from build123d import *

# Parameters (mm, degrees)
SKETCH_1_W             = 85
SKETCH_1_H             = 16
SKETCH_1_R             = 4.25
EXTRUDE_1_DEPTH        = 10
HOLE_WIZARD_M5_1_D     = 4.2
HOLE_WIZARD_M5_1_DEPTH = 14.9
HOLE_WIZARD_M5_1_TIP   = 1.2618073


with BuildPart() as part:
    # 草图1 → 凸台-拉伸1 (new body)
    with BuildSketch(Plane.XY):
        Rectangle(SKETCH_1_W, SKETCH_1_H)
        with Locations((-23, 0)):
            Circle(SKETCH_1_R, mode=Mode.SUBTRACT)
        with Locations((23, 0)):
            Circle(SKETCH_1_R, mode=Mode.SUBTRACT)
    extrude(amount=EXTRUDE_1_DEPTH)

    # M5 螺纹孔1
    with Locations(Plane.XY.offset(10)):
        with Locations((-35, 0), (35, 0)):
            Hole(HOLE_WIZARD_M5_1_D / 2, depth=HOLE_WIZARD_M5_1_DEPTH)
            with Locations((0, 0, -(HOLE_WIZARD_M5_1_DEPTH + HOLE_WIZARD_M5_1_TIP / 2))):  # 118° drill point
                Cone(0, HOLE_WIZARD_M5_1_D / 2, HOLE_WIZARD_M5_1_TIP, mode=Mode.SUBTRACT)


solid = part.part
Read the model definition and answer for the solid it produces. Units are mm, in the model's axes. Give positions to 0.01 mm unless a question says otherwise; leave off trailing zeros. Write each loop counter-clockwise with the first axis right and the second up, starting at its lowest first coordinate (ties: lowest second). Pieces come first, ordered by that corner, then holes. Notation, with made-up numbers: (28, 61.5) -> (44, 61.5) arc R12 ccw to (44, 71.5) -> close; hole circle Ø6 at (69, 34). An arc over 180 degrees is marked (long way). Answer as a JSON object with one key per item and string values. Group by question number.
1) Find section D-D (x = -35). Write down the section's boundary in (y, z), and give its area (3 significant figures).
2) The mould has two halves that part along X. Classify faces 1 (the flat face through (-1, 8, 5)), 2 (the flat face through (42.5, 0, 5)), 3 (the cylindrical face through (19.868, 2.872, 4.93)): +X half, -X half, draft (parallel to the pull), parting line (faces both ways), or undercut.
3) Find section A-A (y = 0). Write down the section's boundary in (x, z).
4) Find section B-B (x = 23). Write down the section's boundary in (y, z).
5) Find section C-C (z = 8.5). Write down the section's boundary in (x, y).
6) Consider L1, parallel to Y at x = 23, z = 2.75; L2, parallel to X at y = 1.25, z = 8; L3, parallel to Y at x = -35, z = 2.75. Determine where each line is inside the solid, lowest interval first. Write a range as from..to.
7) This flat-tipped pin is pushed along its axis until it touches: P1, Ø4, axis at x = -35, y = 0, coming from the -Z side. Where does it stop, or does it pass through?
Values follow:
{
 "1": {"outline": "(-8, 0) -> (-2.1, 0) -> (-2.1, 10) -> (-8, 10) -> close; (2.1, 0) -> (8, 0) -> (8, 10) -> (2.1, 10) -> close", "area": "118 mm2"},
 "2": {"face 1": "draft", "face 2": "+X half", "face 3": "undercut"},
 "3": {"outline": "(-42.5, 0) -> (-37.1, 0) -> (-37.1, 10) -> (-42.5, 10) -> close; (-32.9, 0) -> (-27.25, 0) -> (-27.25, 10) -> (-32.9, 10) -> close; (-18.75, 0) -> (18.75, 0) -> (18.75, 10) -> (-18.75, 10) -> close; (27.25, 0) -> (32.9, 0) -> (32.9, 10) -> (27.25, 10) -> close; (37.1, 0) -> (42.5, 0) -> (42.5, 10) -> (37.1, 10) -> close"},
 "4": {"outline": "(-8, 0) -> (-4.25, 0) -> (-4.25, 10) -> (-8, 10) -> close; (4.25, 0) -> (8, 0) -> (8, 10) -> (4.25, 10) -> close"},
 "5": {"outline": "(-42.5, -8) -> (42.5, -8) -> (42.5, 8) -> (-42.5, 8) -> close; hole circle Ø4.2 at (-35, 0); hole circle Ø8.5 at (-23, 0); hole circle Ø8.5 at (23, 0); hole circle Ø4.2 at (35, 0)"},
 "6": {"L1": "y = -8..-4.25, 4.25..8", "L2": "x = -42.5..-36.69, -33.31..-27.06, -18.94..18.94, 27.06..33.31, 36.69..42.5", "L3": "y = -8..-2.1, 2.1..8"},
 "7": {"P1": "passes through"}
}
